Geometry: final body of the model. Coordinates: model frame, mm. A direction names the side the tool comes from. Give positions to 0.01 mm unless a question says otherwise; leave off trailing zeros. Order: outer loops, then holes, each group sorted by start corner. A loop starts at its lowest first (then second) coordinate and runs counter-clockwise, first axis right, second up. Notation, with made-up numbers: (52.5, 89) -> (67.5, 89) arc R20 ccw to (67.5, 126) -> close; hole circle Ø1 at (60, 16.5). An arc over 180 degrees is marked (long way). Answer in a Markdown table with one row per item. Add a question column.
Q1. Cut plane A-A on y = -19. Return the cut outline in (x, z), and give its area (3 significant figures).
Q2. Cut plane C-C on y = -55.5. Return the cut outline in (x, z).
Q3. Line query: line 1 along X through (y, z) = (-130.5, 97). Output: solid intervals per line, ascending. Write a range as from..to.
Q4. Contact query for flat-ended pins moving along their axis: P1, Ø4, axis at x = -27, y = -33.5, coming from the +Z side; P2, Ø11, axis at y = -129.5, z = -5.5, coming from the +X side; P3, Ø1, axis at x = 35.5, z = 40.5, coming from the -Y side; P4, Ø1.8, axis at y = -93, z = 96.5, coming from the -X side. Output: stop coordinate, or through.
Q5. Cut plane B-B on z = 6.5. Return the cut outline in (x, y).
Q6. Set-up query: faces 1 (the face through (43.27, -149.82, 51.41)), 2 (the face through (-28, -50.8, -5)), 3 (the face through (-28, -28, 0)). Return all of +Z, -Z, +X, -X, +Y, -Y with unobstructed straight access to the full face (end or side cutting, diameter ignored); none if empty.
from build123d import *

# Parameters (mm, degrees)
F1_DEPTH = 5.08
F2_W     = 5.08
F2_H     = 10.16
F3_DEPTH = 45.72
F4_DEPTH = 142.24
F6_DEPTH = 5.08
F7_W     = 5.068376
F7_H     = 10.1649
F8_DEPTH = 50.8


with BuildPart() as f1:
    # F0 (on Front) → F1 (new body)
    with BuildSketch(Plane.XZ):
        Polygon((115.255311, 101.401368), (-30.794689, 0), (-30.794689, -10.16), (-25.714689, -10.16), (-25.714689, 0), (115.255311, 97.874364), align=None)
    extrude(amount=F1_DEPTH)

    # F2 (on face) → F3 (join)
    with BuildSketch(Plane.XZ.offset(5.08)):
        with Locations((-28.254689, -5.08)):
            Rectangle(F2_W, F2_H)
    extrude(amount=F3_DEPTH)

    # F2 (on face) → F4 (join)
    with BuildSketch(Plane.XZ.offset(5.08)):
        Polygon((115.255311, 101.401368), (111.198959, 98.585075), (111.198959, 95.058071), (115.255311, 97.874364), align=None)
    extrude(amount=F4_DEPTH)

    # F5 (on face) → F6 (join)
    with BuildSketch(Plane.XZ.offset(147.32)):
        Polygon((115.255311, 97.874364), (115.255311, 101.401368), (-30.752653, 0), (-30.752653, -10.1649), (-25.684277, -10.1649), (-25.684277, 0), align=None)
    extrude(amount=F6_DEPTH)

    # F7 (on face) → F8 (join)
    with BuildSketch(Plane.XZ.offset(152.4)):
        with Locations((-28.218465, -5.08245)):
            Rectangle(F7_W, F7_H)
    extrude(amount=-F8_DEPTH)


solid = f1.part
Completed:
| question | item | result |
|---|---|---|
| 1 | outline | (-30.79, -10.16) -> (-25.71, -10.16) -> (-25.71, 0) -> (-30.79, 0) -> close; (111.2, 95.06) -> (115.26, 97.87) -> (115.26, 101.4) -> (111.2, 98.59) -> close |
| 1 | area | 65.9 mm² |
| 2 | outline | (111.2, 95.06) -> (115.26, 97.87) -> (115.26, 101.4) -> (111.2, 98.59) -> close |
| 3 | line 1 | x = 111.2..114 |
| 4 | P1 | stops at z = 0 |
| 4 | P2 | stops at x = -25.68 |
| 4 | P3 | passes through |
| 4 | P4 | stops at x = 111.2 |
| 5 | outline | (-21.43, -5.08) -> (-16.35, -5.08) -> (-16.35, 0) -> (-21.43, 0) -> close; (-21.39, -152.4) -> (-16.32, -152.4) -> (-16.32, -147.32) -> (-21.39, -147.32) -> close |
| 6 | face 1 | +Z, -X, +Y, -Y |
| 6 | face 2 | +Z, -Z, +X, -X |
| 6 | face 3 | +Z, +X, -X |
